Geometry: final body of the model. Coordinates: model frame, mm. A direction names the side the tool comes from. Give positions to 0.01 mm unless a question says otherwise; leave off trailing zeros. Loops run counter-clockwise (first coordinate to the right, second up) from the corner with the lowest first, then second, coordinate; pieces in that order, holes last. Notation, with made-up numbers: (84.25, 33) -> (121.25, 33) arc R35 cw to (121.25, 68) -> close; hole circle Ø6 at (79, 17.5). An arc over 180 degrees is marked (long way). Answer in a Markdown table with one row per item. Add a question column.
1) Section query A-A (z = 0). Return the cut outline in (x, y) (3 decimals), plus the area to 3 significant figures.
2) Access query for faces 1 (the cylindrical face through (-1.706, 7.752, 4.115)), 2 (the flat face through (0, 11.7, 0)). Directions: +Z, -Z, +X, -X, +Y, -Y. A direction counts if a zero-diameter tool reaches every point of the face in a straight line with its end or side. Return the directions, or none.
3) Section query B-B (x = 0). Return the cut outline in (y, z) (3 decimals), plus the area to 3 significant figures.
4) Section query C-C (y = 7.5). Return the cut outline in (x, z) (3 decimals).
5) Line query: line 1 (Y direction, x = -2.5, z = 3.5); line 2 (X direction, y = 6.75, z = 1.25); line 3 (Z direction, x = 2, y = 6). Output: solid intervals per line, ascending. Write a range as from..to.
6) First-contact query: P1, Ø2, axis at x = -1.5, y = 2, coming from the -Z side; P2, Ø1.5, axis at y = 7.5, z = 1.5, coming from the -X side. Flat tips, straight axial feed; report the tip coordinate or a pass-through.
Autodesk Fusion 360 part; units mm, degrees
sketch "Sketch1" plane through (0, 0, 0) normal (1, 0, 0) x (0, 1, 0)
  line L0 (0, 0) -> (0, 4.6)
  line L1 (0, 4.6) -> (3.7, 5)
  line L2 (3.7, 5) -> (3.7, 4.455)
  line L3 (3.7, 4.455) -> (11.7, 4.455)
  line L4 (11.7, 4.455) -> (11.7, 0)
  line L5 (11.7, 0) -> (0, 0)
  dimension "d1" = 4.455
  dimension "d2" = 3.7
  dimension "d3" = 5
  dimension "d4" = 4.6
  dimension "d5" = 8
revolve "Revolve1" add sketch "Sketch1" angle 360 about axis through (0, 11.7, 0) along (0, -1, 0)
fillet "Fillet1" radius 0.25 5 faces at (2.1309, 2.8778, 4.4248) (0.4697, 3.7, 4.7831) (0.2221, 6.3667, 4.4495) (0.3414, 11.7, 0.134) (0.0152, 0, -1.4325)
equation "d1 = ( 8.91 / 2 ) * 1 mm"
equation "d4 = ( 9.2 / 2 ) * 1 mm"
Evaluation:
| question | item | result |
|---|---|---|
| 1 | outline | (-4.97, 3.423) -> (-4.624, 0.223) arc R0.25 ccw to (-4.376, 0) -> (4.376, 0) arc R0.25 ccw to (4.624, 0.223) -> (4.97, 3.423) arc R0.25 ccw to (4.722, 3.7) -> (4.705, 3.7) arc R0.25 cw to (4.455, 3.95) -> (4.455, 11.45) arc R0.25 ccw to (4.205, 11.7) -> (-4.205, 11.7) arc R0.25 ccw to (-4.455, 11.45) -> (-4.455, 3.95) arc R0.25 cw to (-4.705, 3.7) -> (-4.722, 3.7) arc R0.25 ccw to start |
| 1 | area | 107 mm² |
| 2 | face 1 | +Y |
| 2 | face 2 | +Z, -Z, +X, -X, +Y |
| 3 | outline | (0, -4.376) arc R0.25 ccw to (0.223, -4.624) -> (3.423, -4.97) arc R0.25 ccw to (3.7, -4.722) -> (3.7, -4.705) arc R0.25 cw to (3.95, -4.455) -> (11.45, -4.455) arc R0.25 ccw to (11.7, -4.205) -> (11.7, 4.205) arc R0.25 ccw to (11.45, 4.455) -> (3.95, 4.455) arc R0.25 cw to (3.7, 4.705) -> (3.7, 4.722) arc R0.25 ccw to (3.423, 4.97) -> (0.223, 4.624) arc R0.25 ccw to (0, 4.376) -> close |
| 3 | area | 107 mm² |
| 4 | outline | circle Ø8.91 at (0, 0) |
| 5 | line 1 | 0..11.68 |
| 5 | line 2 | -4.28..4.28 |
| 5 | line 3 | -3.98..3.98 |
| 6 | P1 | z = -4.83 |
| 6 | P2 | x = -4.39 |
